```python
from build123d import *

# Parameters (mm, degrees)
CROQUIS1_W              = 240
CROQUIS1_H              = 265
SALIENTE_EXTRUIR1_DEPTH = 240
REDONDEO1_R             = 30
REDONDEO2_R             = 30
CROQUIS2_R              = 30.811504022
SALIENTE_EXTRUIR2_DEPTH = 20
VACIADO1_T              = -3


with BuildPart() as part:
    # Croquis1 → Saliente-Extruir1 (new body)
    with BuildSketch(Plane.XZ):
        with Locations((71.623347888, 113.329596413)):
            Rectangle(CROQUIS1_W, CROQUIS1_H)
    extrude(amount=-SALIENTE_EXTRUIR1_DEPTH)

    # Redondeo1
    redondeo1_edges = [part.edges().sort_by_distance(p)[0] for p in [
        (-48.376652112, 120, 245.829596413),
        (191.623347888, 120, 245.829596413),
        (191.623347888, 120, -19.170403587),
        (-48.376652112, 120, -19.170403587),
    ]]
    fillet(redondeo1_edges, radius=REDONDEO1_R)

    # Redondeo2
    redondeo2_edges = [part.edges().sort_by_distance(p)[0] for p in [
        (71.623347888, 0, -19.170403587),
        (71.623347888, 240, -19.170403587),
        (-48.376652112, 0, 113.329596413),
        (191.623347888, 0, 113.329596413),
        (71.623347888, 0, 245.829596413),
        (-39.589855548, 0, 237.042799848),
        (-39.589855548, 0, -10.383607023),
        (182.836551323, 0, 237.042799848),
        (182.836551323, 0, -10.383607023),
        (191.623347888, 240, 113.329596413),
        (-48.376652112, 240, 113.329596413),
        (71.623347888, 240, 245.829596413),
        (-39.589855548, 240, 237.042799848),
        (-39.589855548, 240, -10.383607023),
        (182.836551323, 240, 237.042799848),
        (182.836551323, 240, -10.383607023),
    ]]
    fillet(redondeo2_edges, radius=REDONDEO2_R)

    # Croquis2 → Saliente-Extruir2 (add)
    with BuildSketch(Plane(origin=(0, 240, 0), x_dir=(1, 0, 0), z_dir=(0, 1, 0))):
        with Locations(Location((70.222158981, -176.211697137, 0), (0, 0, 90))):
            Circle(CROQUIS2_R)
    extrude(amount=SALIENTE_EXTRUIR2_DEPTH)

    # Vaciado1
    vaciado1_openings = [part.faces().sort_by_distance(p)[0] for p in [
        (70.222158981, 260, 176.211697137),
    ]]
    offset(amount=VACIADO1_T, openings=vaciado1_openings, kind=Kind.INTERSECTION)


solid = part.part
```
Check sheet for the modelled part. Datum: model origin and axes. Units: mm. A direction names the side the tool comes from. Give positions to 0.01 mm unless a question says otherwise; leave off trailing zeros. Loops run counter-clockwise (first coordinate to the right, second up) from the corner with the lowest first, then second, coordinate; pieces in that order, holes last. Notation, with made-up numbers: (35.25, 48) - (63.25, 48) arc R12 ccw to (63.25, 53) - close; hole circle Ø9 at (-35, 38). An arc over 180 degrees is marked (long way). One line per question, with ' | ' between items. Start each with the question number.
1. Gauge pin test, flat ends, axial feed: pin 1 Ø2 at (x, z) = (165, 101) entering from +Y; pin 2 Ø10 at (x, z) = (-23.5, 199) entering from +Y. Record the tip position at first contact, or that the pin passes through.
2. Cross-section at B-B, the plane z = 132. Enter the section's corners in (x, y), plus the area to 3 significant figures.
3. Set-up check for faces 5 (the flat face through (-48.377, 119, 112)), 6 (the cylindrical face through (-37.68, 121.26, -8.05)): record each of +Z, -Z, +X, -X, +Y, -Y from which the full face is reachable in a straight line by a thin tool's end or side.
4. Draft check along Z on faces 1 (the cylindrical face through (-39.82, 121.26, 236.81)), 2 (the cylindrical face through (69, 250, 207)), 3 (the cylindrical face through (180.924, 121.26, 234.71)), 4 (the cylindrical face through (-39.4, 8.6, 111.9)). Enter one of: released by +Z, released by -Z, zero draft, split by the parting line, or undercut.
5. Material ranges on line 1 along X through (y, z) = (115.5, 149.5); line 2 along Y through (x, z) = (53, 89); line 3 along Z through (x, y) = (40, 55), recorded low to high. Write a range as [from, to].
6. Cross-section at A-A, the plane x = 15. Enter the section's corners in (y, z).
Check result:
1) pin 1: stops at y = 239.91 | pin 2: stops at y = 240
2) outline: (-48.38, 30) arc R30 ccw to (-18.38, 0) - (161.62, 0) arc R30 ccw to (191.62, 30) - (191.62, 210) arc R30 ccw to (161.62, 240) - (-18.38, 240) arc R30 ccw to (-48.38, 210) - close; hole (-45.38, 30) arc R27 ccw to (-18.38, 3) - (161.62, 3) arc R27 ccw to (188.62, 30) - (188.62, 210) arc R27 ccw to (161.62, 237) - (-18.38, 237) arc R27 ccw to (-45.38, 210) - close | area: 2,700 mm2
3) face 5: +Z, -Z, -X, +Y, -Y | face 6: none
4) face 1: released by +Z | face 2: split by the parting line | face 3: undercut | face 4: zero draft
5) line 1: x = [-48.38, -45.38], [188.62, 191.62] | line 2: y = [0, 3], [237, 240] | line 3: z = [-19.17, -16.17], [242.83, 245.83]
6) outline: (0, 10.83) arc R30 ccw to (30, -19.17) - (210, -19.17) arc R30 ccw to (240, 10.83) - (240, 215.83) arc R30 ccw to (210, 245.83) - (30, 245.83) arc R30 ccw to (0, 215.83) - close; hole (3, 10.83) arc R27 ccw to (30, -16.17) - (210, -16.17) arc R27 ccw to (237, 10.83) - (237, 215.83) arc R27 ccw to (210, 242.83) - (30, 242.83) arc R27 ccw to (3, 215.83) - close
